from build123d import *

# Parameters (mm, degrees)
SKETCH1_W           = 39.899654891
SKETCH1_H           = 96.899161878
BOSS_EXTRUDE1_DEPTH = 25
FILLET4_R           = 4
FILLET5_R           = 4
SKETCH11_R          = 0.836574299
SKETCH11_W          = 1.425486882
SKETCH11_H          = 1.295897166
BOSS_EXTRUDE2_DEPTH = 0.5


with BuildPart() as part:
    # Sketch1 → Boss-Extrude1 (new body)
    with BuildSketch(Plane(origin=(0, 0, 0), x_dir=(1, 0, 0), z_dir=(0, 1, 0))):
        with Locations((-40.909991022, 17.297585728)):
            Rectangle(SKETCH1_W, SKETCH1_H)
    extrude(amount=BOSS_EXTRUDE1_DEPTH)

    # Fillet4
    fillet4_edges = [part.edges().sort_by_distance(p)[0] for p in [
        (-20.960163576, 25, -17.297585728),
        (-40.909991022, 25, -65.747166667),
        (-60.859818467, 25, -17.297585728),
        (-40.909991022, 0, -65.747166667),
        (-20.960163576, 0, -17.297585728),
        (-40.909991022, 0, 31.151995211),
        (-60.859818467, 0, -17.297585728),
        (-40.909991022, 25, 31.151995211),
    ]]
    fillet(fillet4_edges, radius=FILLET4_R)

    # Fillet5
    # the kernel refuses this fillet: 4 mm, written as the material it takes off along each edge
    with BuildSketch(Plane(origin=(-56.859818467, 4, -61.747166667), x_dir=(-1, 0, 0), z_dir=(0, 0, -1))) as fillet5_piece_1_section:
        Polygon((0, 0), (FILLET5_R, 0), (FILLET5_R, -FILLET5_R), (0, -FILLET5_R), align=None)
    fillet5_piece_1 = extrude(amount=FILLET5_R, mode=Mode.PRIVATE)
    fillet5_piece_1 = fillet5_piece_1 - Plane(origin=(-56.859818467, 4, -61.747166667), x_dir=(0.7071067811865475, 0.7071067811865475, 0), z_dir=(0, 0, -1)) * Sphere(FILLET5_R, mode=Mode.PRIVATE)
    add(fillet5_piece_1, mode=Mode.SUBTRACT)
    with BuildSketch(Plane(origin=(-24.960163576, 4, -61.747166667), x_dir=(1, 0, 0), z_dir=(0, 0, -1))) as fillet5_piece_2_section:
        Polygon((0, 0), (FILLET5_R, 0), (FILLET5_R, FILLET5_R), (0, FILLET5_R), align=None)
    fillet5_piece_2 = extrude(amount=FILLET5_R, mode=Mode.PRIVATE)
    fillet5_piece_2 = fillet5_piece_2 - Plane(origin=(-24.960163576, 4, -61.747166667), x_dir=(-0.7071067811865475, 0.7071067811865475, 0), z_dir=(0, 0, -1)) * Sphere(FILLET5_R, mode=Mode.PRIVATE)
    add(fillet5_piece_2, mode=Mode.SUBTRACT)
    with BuildSketch(Plane(origin=(-56.859818467, 4, 27.151995211), x_dir=(0, 0, 1), z_dir=(-1, 0, 0))) as fillet5_piece_3_section:
        Polygon((0, 0), (FILLET5_R, 0), (FILLET5_R, -FILLET5_R), (0, -FILLET5_R), align=None)
    fillet5_piece_3 = extrude(amount=FILLET5_R, mode=Mode.PRIVATE)
    fillet5_piece_3 = fillet5_piece_3 - Plane(origin=(-56.859818467, 4, 27.151995211), x_dir=(0, 0.7071067811865475, -0.7071067811865475), z_dir=(-1, 0, 0)) * Sphere(FILLET5_R, mode=Mode.PRIVATE)
    add(fillet5_piece_3, mode=Mode.SUBTRACT)
    with BuildSketch(Plane(origin=(-24.960163576, 4, 27.151995211), x_dir=(0, 0, 1), z_dir=(1, 0, 0))) as fillet5_piece_4_section:
        Polygon((0, 0), (FILLET5_R, 0), (FILLET5_R, FILLET5_R), (0, FILLET5_R), align=None)
    fillet5_piece_4 = extrude(amount=FILLET5_R, mode=Mode.PRIVATE)
    fillet5_piece_4 = fillet5_piece_4 - Plane(origin=(-24.960163576, 4, 27.151995211), x_dir=(0, 0.7071067811865475, -0.7071067811865475), z_dir=(1, 0, 0)) * Sphere(FILLET5_R, mode=Mode.PRIVATE)
    add(fillet5_piece_4, mode=Mode.SUBTRACT)
    with BuildSketch(Plane(origin=(-24.960163576, 21, 27.151995211), x_dir=(0, 0, 1), z_dir=(1, 0, 0))) as fillet5_piece_5_section:
        Polygon((0, 0), (FILLET5_R, 0), (FILLET5_R, -FILLET5_R), (0, -FILLET5_R), align=None)
    fillet5_piece_5 = extrude(amount=FILLET5_R, mode=Mode.PRIVATE)
    fillet5_piece_5 = fillet5_piece_5 - Plane(origin=(-24.960163576, 21, 27.151995211), x_dir=(0, -0.7071067811865475, -0.7071067811865475), z_dir=(1, 0, 0)) * Sphere(FILLET5_R, mode=Mode.PRIVATE)
    add(fillet5_piece_5, mode=Mode.SUBTRACT)
    with BuildSketch(Plane(origin=(-56.859818467, 21, 27.151995211), x_dir=(0, 0, 1), z_dir=(-1, 0, 0))) as fillet5_piece_6_section:
        Polygon((0, 0), (FILLET5_R, 0), (FILLET5_R, FILLET5_R), (0, FILLET5_R), align=None)
    fillet5_piece_6 = extrude(amount=FILLET5_R, mode=Mode.PRIVATE)
    fillet5_piece_6 = fillet5_piece_6 - Plane(origin=(-56.859818467, 21, 27.151995211), x_dir=(0, -0.7071067811865475, -0.7071067811865475), z_dir=(-1, 0, 0)) * Sphere(FILLET5_R, mode=Mode.PRIVATE)
    add(fillet5_piece_6, mode=Mode.SUBTRACT)
    with BuildSketch(Plane(origin=(-24.960163576, 21, -61.747166667), x_dir=(1, 0, 0), z_dir=(0, 0, -1))) as fillet5_piece_7_section:
        Polygon((0, 0), (FILLET5_R, 0), (FILLET5_R, -FILLET5_R), (0, -FILLET5_R), align=None)
    fillet5_piece_7 = extrude(amount=FILLET5_R, mode=Mode.PRIVATE)
    fillet5_piece_7 = fillet5_piece_7 - Plane(origin=(-24.960163576, 21, -61.747166667), x_dir=(-0.7071067811865475, -0.7071067811865475, 0), z_dir=(0, 0, -1)) * Sphere(FILLET5_R, mode=Mode.PRIVATE)
    add(fillet5_piece_7, mode=Mode.SUBTRACT)
    with BuildSketch(Plane(origin=(-56.859818467, 21, -61.747166667), x_dir=(-1, 0, 0), z_dir=(0, 0, -1))) as fillet5_piece_8_section:
        Polygon((0, 0), (FILLET5_R, 0), (FILLET5_R, FILLET5_R), (0, FILLET5_R), align=None)
    fillet5_piece_8 = extrude(amount=FILLET5_R, mode=Mode.PRIVATE)
    fillet5_piece_8 = fillet5_piece_8 - Plane(origin=(-56.859818467, 21, -61.747166667), x_dir=(0.7071067811865475, -0.7071067811865475, 0), z_dir=(0, 0, -1)) * Sphere(FILLET5_R, mode=Mode.PRIVATE)
    add(fillet5_piece_8, mode=Mode.SUBTRACT)
    with BuildSketch(Plane(origin=(-20.960163576, 4, 31.151995211), x_dir=(0, 0, -1), z_dir=(0, 1, 0)), Plane(origin=(-20.960163576, 4, -65.747166667), x_dir=(-1, 0, 0), z_dir=(0, 1, 0))) as fillet5_piece_9:
        with BuildLine():
            CenterArc((FILLET5_R, FILLET5_R), FILLET5_R, 180, 90)
            Line((0, FILLET5_R), (0, 0))
            Line((0, 0), (FILLET5_R, 0))
        make_face()
    extrude(amount=17, mode=Mode.SUBTRACT)
    with BuildSketch(Plane(origin=(-60.859818467, 4, 31.151995211), x_dir=(0, 0, -1), z_dir=(0, 1, 0)), Plane(origin=(-60.859818467, 4, -65.747166667), x_dir=(1, 0, 0), z_dir=(0, 1, 0))) as fillet5_piece_10:
        with BuildLine():
            CenterArc((FILLET5_R, -FILLET5_R), FILLET5_R, 90, 90)
            Line((0, -FILLET5_R), (0, 0))
            Line((0, 0), (FILLET5_R, 0))
        make_face()
    extrude(amount=17, mode=Mode.SUBTRACT)

    # Sketch11 → Boss-Extrude2 (add)
    with BuildSketch(Plane.XY.offset(31.151995211)):
        with Locations(Location((-29.976452447, 19.823866424, 0), (0, 0, 180))):
            Circle(SKETCH11_R)
        with Locations(Location((-29.976452447, 17.95408771, 0), (0, 0, 180))):
            Circle(SKETCH11_R)
        with Locations(Location((-29.976452447, 14.298065843, 0), (0, 0, 180))):
            Circle(SKETCH11_R)
        with Locations(Location((-29.976452447, 16.144719304, 0), (0, 0, 180))):
            Circle(SKETCH11_R)
        with Locations((-53.429405659, 5.097195967)):
            Rectangle(SKETCH11_W, SKETCH11_H)
        with Locations((-53.429405659, 6.943849428)):
            Rectangle(SKETCH11_W, SKETCH11_H)
    extrude(amount=BOSS_EXTRUDE2_DEPTH)


solid = part.part
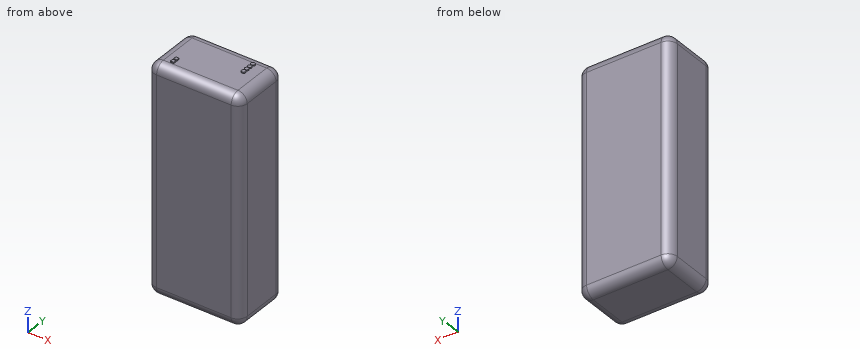
CAD build for the part. Positions are in the model's coordinates, mm. Give positions to 0.01 mm unless a question says otherwise; leave off trailing zeros. Order: outer loops, then holes, each group sorted by start corner. A loop starts at its lowest first (then second) coordinate and runs counter-clockwise, first axis right, second up. Notation, with made-up numbers: (35, 54.25) - (88, 54.25) arc R23 ccw to (88, 79.25) - close; hole circle Ø10 at (4.5, 74.5). An arc over 180 degrees is marked (long way). Answer in a Markdown table with one row per item.
1. Saw through at A-A, the plane x = -58. Give the cut face in (y, z).
Data:
| item | result |
|---|---|
| outline | (0.17, -61.75) arc R3.83 ccw to (4, -65.58) - (21, -65.58) arc R3.83 ccw to (24.83, -61.75) - (24.83, 27.15) arc R3.83 ccw to (21, 30.99) - (4, 30.99) arc R3.83 ccw to (0.17, 27.15) - close |
2. Flat gauge pins, fed straight in: pin 1 (0.6 mm diameter, centred on y = 7, z = 31.5, fed in from -X); pin 2 (1.5 mm diameter, centred on x = -41, y = 9, fed in from +Z). Where does each tip first touch, or does it go through?
Data:
| item | result |
|---|---|
| pin 1 | stops at x = -54.14 |
| pin 2 | stops at z = 31.15 |
3. Saw through at B-B, the plane y = 23. Give the cut face in (x, z), plus the area to 3 significant figures.
Data:
| item | result |
|---|---|
| outline | (-60.32, -61.75) arc R3.46 ccw to (-56.86, -65.21) - (-24.96, -65.21) arc R3.46 ccw to (-21.5, -61.75) - (-21.5, 27.15) arc R3.46 ccw to (-24.96, 30.62) - (-56.86, 30.62) arc R3.46 ccw to (-60.32, 27.15) - close |
| area | 3,710 mm² |
4. Probe probe 1 along Z at (x, y) = (-33.5, 13.5); probe 2 along X at (y, z) = (21.25, -61); probe 3 along X at (y, z) = (19.75, 27.5). List the from-to ranges inside material, lowest first. Write a range as [from, to].
Data:
| item | result |
|---|---|
| probe 1 | z = [-65.75, 31.15] |
| probe 2 | x = [-60.85, -20.97] |
| probe 3 | x = [-60.84, -20.98] |
